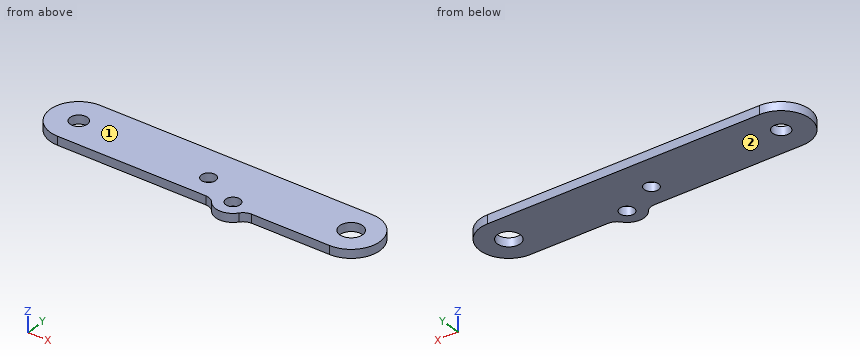
Autodesk Inventor part; units mm, degrees
ref_plane "YZ Plane" through (0, 0, 0) normal (1, 0, 0) x (0, 1, 0)
ref_plane "XZ Plane" through (0, 0, 0) normal (0, 1, 0) x (-1, 0, 0)
ref_plane "XY Plane" through (0, 0, 0) normal (0, 0, 1) x (1, 0, 0)
sketch "Szkic1" plane through (0, 0, 0) normal (0, 0, 1) x (1, 0, 0)
  line L0 (0, 0) -> (95, 0) construction
  line L1 (0, -10) -> (5.8348, -10)
  line L2 (95, 10) -> (0, 10)
  arc A0 (0, 10) -> (0, -10) centre (0, 0) ccw
  arc A1 (95, -10) -> (95, 10) centre (95, 0) ccw
  line L3 (5.8348, -10) -> (51.7624, -10)
  arc A2 (54.9624, -11.6) -> (64.5624, -11.6) centre (59.7624, -8) ccw
  line L4 (67.7624, -10) -> (95, -10)
  arc A3 (54.9624, -11.6) -> (51.7624, -10) centre (51.7624, -14) ccw
  arc A4 (67.7624, -10) -> (64.5624, -11.6) centre (67.7624, -14) ccw
  point P0 (47.5, 0)
  point P1 (46.7624, -2)
  point P2 (65.4193, -10)
  point P3 (54.1056, -10)
  point P4 (54.7624, -1)
  dimension "d0" = 95
  dimension "d1" = 20
  dimension "d23" = 12
  dimension "d24" = 4
  dimension "d34" = 8
  dimension "d35" = 5
  dimension "d36" = 7
  dimension "d37" = 1
  dimension "d38" = 6
  dimension "d40" = 40.25
  dimension "d41" = 1
extrude "Wyciągnięcie proste1" add sketch "Szkic1" along normal blind 3
hole "Otwór1" at (95, 0, 0) direction (0, 0, 1) diameter 8 end through all
hole "Otwór2" at (46.7624, -2, 0) at (59.7624, -8, 0) direction (0, 0, 1) diameter 5 end through all
hole "Otwór3" at (0, 0, 0) direction (0, 0, 1) diameter 6 end through all
properties part number "ramie_napinacza"
Part model, mm, in its own coordinate system. Face numbers are marked on the shaded views. Round coordinates to 2 decimals unless told otherwise and drop trailing zeros. Write each loop counter-clockwise with the first axis right and the second up, starting at its lowest first coordinate (ties: lowest second). Pieces come first, ordered by that corner, then holes. Notation, with made-up numbers: (86.25, 76.25) - (127.25, 76.25) arc R31 cw to (127.25, 112.25) - close; hole circle Ø5 at (77.5, 9). An arc over 180 degrees is marked (long way). Use CSV: the item, a comma, the result in double quotes.
Item 1: Wall check: L1, parallel to X at y = 0, z = 1.3; L2, parallel to X at y = -2, z = 0.95; L3, parallel to X at y = 1, z = 2.3. Give the ranges that are in metal, low to high.
Results list:
L1,"x = -10 to -3, 3 to 45.26, 48.26 to 91, 99 to 105"
L2,"x = -9.8 to -2.24, 2.24 to 44.26, 49.26 to 91.54, 98.46 to 104.8"
L3,"x = -9.95 to -2.83, 2.83 to 91.13, 98.87 to 104.95"
Item 2: Flat gauge pins, fed straight in: P1, Ø1.5, axis at x = 28.5, z = 2, coming from the -Y side; P2, Ø3, axis at x = 46.76, y = -2, coming from the +Z side; P3, Ø1.5, axis at y = 3, z = 2, coming from the +X side. Where does each tip first touch, or does it go through?
Results list:
P1,"stops at y = -10"
P2,"passes through"
P3,"stops at x = 104.74"
Item 3: Slice it at B-B, the plane z = 0.5. Write the cut outline in (x, y), then the cut area to 3 significant figures.
Results list:
outline,"(0, -10) - (51.76, -10) arc R4 cw to (54.96, -11.6) arc R6 ccw to (64.56, -11.6) arc R4 cw to (67.76, -10) - (95, -10) arc R10 ccw to (95, 10) - (0, 10) arc R10 ccw to start; hole circle Ø6 at (0, 0); hole circle Ø5 at (46.76, -2); hole circle Ø5 at (59.76, -8); hole circle Ø8 at (95, 0)"
area,"2,130 mm²"
Item 4: Slice it at D-D, the plane x = 25.5. Write the cut outline in (y, z).
Results list:
outline,"(-10, 0) - (10, 0) - (10, 3) - (-10, 3) - close"
Item 5: Slice it at C-C, the plane y = -2. Write the cut outline in (x, z), then the cut area to 3 significant figures.
Results list:
outline,"(-9.8, 0) - (-2.24, 0) - (-2.24, 3) - (-9.8, 3) - close; (2.24, 0) - (44.26, 0) - (44.26, 3) - (2.24, 3) - close; (49.26, 0) - (91.54, 0) - (91.54, 3) - (49.26, 3) - close; (98.46, 0) - (104.8, 0) - (104.8, 3) - (98.46, 3) - close"
area,"295 mm²"
Item 6: Slice it at A-A, the plane y = -8. Write the cut outline in (x, z), then the cut area to 3 significant figures.
Results list:
outline,"(-6, 0) - (57.26, 0) - (57.26, 3) - (-6, 3) - close; (62.26, 0) - (101, 0) - (101, 3) - (62.26, 3) - close"
area,"306 mm²"
Item 7: Pull direction Z, two halves, no side cores. Call the marked faces 1 and 2: pulls with the +Z half, pulls with the -Z half, needs draft (parallel to the pull), parting line crosses it, or undercut.
Results list:
face 1,"pulls with the +Z half"
face 2,"pulls with the -Z half"
